from build123d import *

# Parameters (mm, degrees)
F1_DEPTH = 63.5
F2_W     = 44.45
F2_H     = 25.4
F3_DEPTH = 63.5


with BuildPart() as f1:
    # F0 (on Front) → F1 (new body)
    with BuildSketch(Plane.XZ):
        Polygon((-41.275, 31.75), (-41.275, -31.75), (41.275, -31.75), (85.725, -31.75), (85.725, -12.7), (41.275, -12.7), (41.275, 31.75), align=None)
    extrude(amount=F1_DEPTH)

    # F2 (on face) → F3 (cut)
    with BuildSketch(Plane.XY.offset(31.75)):
        with Locations((0, -31.75)):
            Rectangle(F2_W, F2_H)
    extrude(amount=-F3_DEPTH, mode=Mode.SUBTRACT)


solid = f1.part
CAD build for the part. Positions are in the model's coordinates, mm. A direction names the side the tool comes from. Coordinates: 2 decimals unless noted, no trailing zeros. Loops run counter-clockwise (first coordinate to the right, second up) from the corner with the lowest first, then second, coordinate; pieces in that order, holes last. Notation, with made-up numbers: (39, -20) -> (63, -20) arc R19 ccw to (63, -5) -> close; hole circle Ø7 at (18.25, 10). An arc over 180 degrees is marked (long way). One line per item, written item: value.
1. Flat gauge pins, fed straight in: P1, Ø22, axis at x = 70.5, y = -18.5, coming from the +Z side; P2, Ø5, axis at y = -31, z = 14, coming from the +X side (3 decimals). Where does each tip first touch, or does it go through?
Answers:
P1: stops at z = -12.7
P2: stops at x = 41.275
2. Slice it at C-C on z = 16.5. Write the cut outline in (x, y) (3 decimals).
Answers:
outline: (-41.275, -63.5) -> (41.275, -63.5) -> (41.275, 0) -> (-41.275, 0) -> close; hole (-22.225, -44.45) -> (22.225, -44.45) -> (22.225, -19.05) -> (-22.225, -19.05) -> close
3. Slice it at D-D on y = -51. Write the cut outline in (x, z) (3 decimals), and give its area (3 significant figures).
Answers:
outline: (-41.275, -31.75) -> (85.725, -31.75) -> (85.725, -12.7) -> (41.275, -12.7) -> (41.275, 31.75) -> (-41.275, 31.75) -> close
area: 6,090 mm^2
4. Pull direction X, two halves, no side cores. Call faces 4 (the face through (0, -19.05, 0)), 5 (the face through (35, -31, -31.75)), 6 (the face through (-22.225, -32, 0)), 7 (the face through (85.725, -31, -22)): pulls with the +X half, pulls with the -X half, needs draft (parallel to the pull), parting line crosses it, or undercut.
Answers:
face 4: undercut
face 5: needs draft
face 6: undercut
face 7: pulls with the +X half
5. Slice it at A-A on x = 10.5. Write the cut outline in (y, z), and give its area (3 significant figures).
Answers:
outline: (-63.5, -31.75) -> (-44.45, -31.75) -> (-44.45, 31.75) -> (-63.5, 31.75) -> close; (-19.05, -31.75) -> (0, -31.75) -> (0, 31.75) -> (-19.05, 31.75) -> close
area: 2,420 mm^2
6. Which spindle directions (+Z, -Z, +X, -X, +Y, -Y) get a long thin tool onto all of the face, cutting with end or side? Do faces 1 (the face through (64, -31, -12.7)), 2 (the face through (22.225, -32, 0)), 3 (the face through (-41.275, -31, 0)). Say none if no direction does.
Answers:
face 1: +Z, +X, +Y, -Y
face 2: +Z, -Z
face 3: +Z, -Z, -X, +Y, -Y
7. Drill centre lines: line 1 (Y direction, x = -22, z = -8); line 2 (X direction, y = -30.5, z = -8) (3 decimals); line 3 (Z direction, x = 80, y = -20.5). Where is each one in solid material? Low to high. Write a range as [from, to].
Answers:
line 1: y = [-63.5, -44.45], [-19.05, 0]
line 2: x = [-41.275, -22.225], [22.225, 41.275]
line 3: z = [-31.75, -12.7]
8. Slice it at B-B on y = -22. Write the cut outline in (x, z) (3 decimals).
Answers:
outline: (-41.275, -31.75) -> (-22.225, -31.75) -> (-22.225, 31.75) -> (-41.275, 31.75) -> close; (22.225, -31.75) -> (85.725, -31.75) -> (85.725, -12.7) -> (41.275, -12.7) -> (41.275, 31.75) -> (22.225, 31.75) -> close
